Part model, mm, in its own coordinate system. Coordinates: 2 decimals unless noted, no trailing zeros. Loops run counter-clockwise (first coordinate to the right, second up) from the corner with the lowest first, then second, coordinate; pieces in that order, holes last.
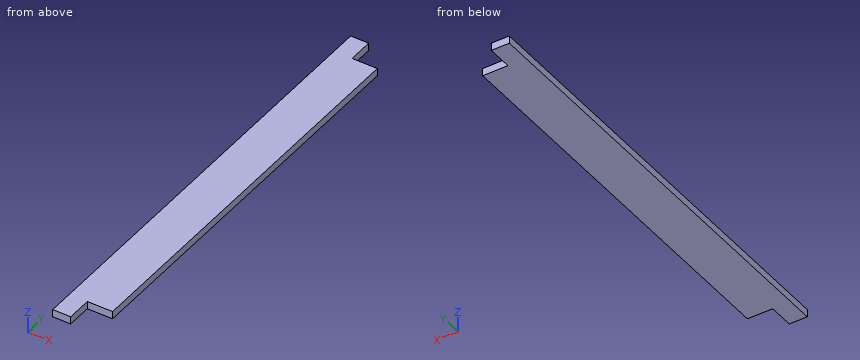
```python
from build123d import *

# Parameters (mm, degrees)
F0_W     = 120
F0_H     = 21
F1_DEPTH = 1255
F2_W     = 70
F2_H     = 70
F3_DEPTH = 25


with BuildPart() as f1:
    # F0 (on Front) → F1 (new body)
    with BuildSketch(Plane.XZ):
        Rectangle(F0_W, F0_H)
    extrude(amount=F1_DEPTH)

    # F2 (on face) → F3 (cut)
    with BuildSketch(Plane.XY.offset(10.5)):
        with Locations((25, -1220)):
            Rectangle(F2_W, F2_H)
        with Locations((25, -35)):
            Rectangle(F2_W, F2_H)
    extrude(amount=-F3_DEPTH, mode=Mode.SUBTRACT)


with BuildPart() as f4_1:
    # F4: copy of F1
    add(f1.part)


solid = f4_1.part
```
Q1. Drop flat-ended pins along their axis: P1, Ø3, axis at x = -15.5, z = 4.5, coming from the +Y side; P2, Ø10.5, axis at x = 20, z = -1.5, coming from the -Y side; P3, Ø4, axis at x = 31.5, z = -6, coming from the +Y side. Give the stop position or say it passes through.
Q2. Saw through at A-A (z = -4.75). List the corners of the cut face in (x, y).
Q3. Probe line 1 (Y direction, x = 3, z = -0.25). List the from-to ranges inside material, lowest first.
Q4. Saw through at B-B (x = 12). List the corners of the cut face in (y, z).
Checked values:
1. P1: stops at y = 0
1. P2: stops at y = -1185
1. P3: stops at y = -70
2. outline: (-60, -1255) - (-10, -1255) - (-10, -1185) - (60, -1185) - (60, -70) - (-10, -70) - (-10, 0) - (-60, 0) - close
3. line 1: y = -1185 to -70
4. outline: (-1185, -10.5) - (-70, -10.5) - (-70, 10.5) - (-1185, 10.5) - close
